```python
from build123d import *

# Parameters (mm, degrees)
SKETCH1_W                   = 38.1
SKETCH1_H                   = 25.4
BOSS_EXTRUDE1_DEPTH         = 25.4
SKETCH3_R                   = 1.5875
CUT_EXTRUDE2_DEPTH          = 25.4
F_1_4_28_TAPPED_HOLE1_D     = 5.4102
F_1_4_28_TAPPED_HOLE1_DEPTH = 17.23
F_1_4_28_TAPPED_HOLE1_TIP   = 1.625388061
SKETCH2_R                   = 3.18
CUT_EXTRUDE6_DEPTH          = 15.875
SKETCH8_R                   = 1.5875
CUT_EXTRUDE7_DEPTH          = 35.1957966
SKETCH9_W                   = 19.05
SKETCH9_H                   = 25.4
BOSS_EXTRUDE2_DEPTH         = 12.7
SKETCH12_W                  = 38.05497839
SKETCH12_H                  = 25.4
BOSS_EXTRUDE3_DEPTH         = 44.45
CUT_EXTRUDE8_START          = -44.45
SKETCH14_R                  = 1.5875
CUT_EXTRUDE8_DEPTH          = 44.45
F_1_4_28_TAPPED_HOLE2_D     = 5.4102
F_1_4_28_TAPPED_HOLE2_DEPTH = 17.23
F_1_4_28_TAPPED_HOLE2_TIP   = 1.625388061
BOSS_EXTRUDE6_DEPTH         = 34.925


with BuildPart() as part:
    # Sketch1 → Boss-Extrude1 (new body)
    with BuildSketch(Plane(origin=(0, 0, 0), x_dir=(1, 0, 0), z_dir=(0, 1, 0))):
        Rectangle(SKETCH1_W, SKETCH1_H)
    extrude(amount=BOSS_EXTRUDE1_DEPTH)

    # Sketch3 → Cut-Extrude2 (cut)
    with BuildSketch(Plane.ZY.offset(19.05)):
        with Locations((0, 12.7)):
            Circle(SKETCH3_R)
    extrude(amount=-CUT_EXTRUDE2_DEPTH, mode=Mode.SUBTRACT)

    # 1/4-28 Tapped Hole1
    with Locations(Plane.ZY.offset(19.05)):
        with Locations((0, 12.7)):
            Hole(F_1_4_28_TAPPED_HOLE1_D / 2, depth=F_1_4_28_TAPPED_HOLE1_DEPTH)
            with Locations((0, 0, -(F_1_4_28_TAPPED_HOLE1_DEPTH + F_1_4_28_TAPPED_HOLE1_TIP / 2))):  # 118° drill point
                Cone(0, F_1_4_28_TAPPED_HOLE1_D / 2, F_1_4_28_TAPPED_HOLE1_TIP, mode=Mode.SUBTRACT)

    # Sketch2 → Cut-Extrude6 (cut)
    with BuildSketch(Plane(origin=(0, 25.4, 0), x_dir=(1, 0, 0), z_dir=(0, 1, 0))):
        with Locations(Location((6.35, 0, 0), (0, 0, 270))):
            Circle(SKETCH2_R)
    extrude(amount=-CUT_EXTRUDE6_DEPTH, mode=Mode.SUBTRACT)

    # Sketch8 → Cut-Extrude7 (cut, through all)
    with BuildSketch(Plane.XZ):
        with Locations(Location((6.35, 0, 0), (0, 0, 270))):
            Circle(SKETCH8_R)
    extrude(amount=-CUT_EXTRUDE7_DEPTH, mode=Mode.SUBTRACT)

    # Sketch9 → Boss-Extrude2 (add)
    with BuildSketch(Plane.XZ):
        with Locations((-9.525, 0)):
            Rectangle(SKETCH9_W, SKETCH9_H)
    extrude(amount=BOSS_EXTRUDE2_DEPTH)

    # Sketch12 → Boss-Extrude3 (add)
    with BuildSketch(Plane.XZ.offset(12.7)):
        with Locations((-0.022510805, 0)):
            Rectangle(SKETCH12_W, SKETCH12_H)
    extrude(amount=BOSS_EXTRUDE3_DEPTH)

    # Sketch14 → Cut-Extrude8 (cut)
    with BuildSketch(Plane(origin=(0, -12.7, 0), x_dir=(1, 0, 0), z_dir=(0, 1, 0)).offset(CUT_EXTRUDE8_START)):
        with Locations(Location((6.35, 0, 0), (0, 0, 90))):
            Circle(SKETCH14_R)
    extrude(amount=CUT_EXTRUDE8_DEPTH, mode=Mode.SUBTRACT)

    # 1/4-28 Tapped Hole2
    with Locations(Plane(origin=(0, -57.15, 0), x_dir=(-1, 0, 0), z_dir=(0, -1, 0))):
        with Locations((-6.35, 0)):
            Hole(F_1_4_28_TAPPED_HOLE2_D / 2, depth=F_1_4_28_TAPPED_HOLE2_DEPTH)
            with Locations((0, 0, -(F_1_4_28_TAPPED_HOLE2_DEPTH + F_1_4_28_TAPPED_HOLE2_TIP / 2))):  # 118° drill point
                Cone(0, F_1_4_28_TAPPED_HOLE2_D / 2, F_1_4_28_TAPPED_HOLE2_TIP, mode=Mode.SUBTRACT)

    # Sketch24 → Boss-Extrude6 (add)
    with BuildSketch(Plane(origin=(0, 25.4, 0), x_dir=(1, 0, 0), z_dir=(0, 1, 0))):
        with BuildLine():
            Line((6.35, -3.302), (19.05, -3.302))
            Line((19.05, -3.302), (19.05, -12.7))
            Line((19.05, -12.7), (-19.05, -12.7))
            Line((-19.05, -12.7), (-19.05, 12.7))
            Line((-19.05, 12.7), (19.05, 12.7))
            Line((19.05, 12.7), (19.05, 3.302))
            Line((19.05, 3.302), (6.35, 3.302))
            ThreePointArc((6.35, 3.302), (3.048, 0), (6.35, -3.302))
        make_face()
    extrude(amount=BOSS_EXTRUDE6_DEPTH)


solid = part.part
```
The model under review builds one solid part; all positions refer to its coordinate system, in mm. A direction names the side the tool comes from. Round coordinates to 2 decimals unless told otherwise and drop trailing zeros. Order: outer loops, then holes, each group sorted by start corner. A loop starts at its lowest first (then second) coordinate and runs counter-clockwise, first axis right, second up. Notation, with made-up numbers: (25, 50) -> (29, 50) arc R27 ccw to (29, 86) -> close; hole circle Ø7 at (-31.75, 64). An arc over 180 degrees is marked (long way). One line per item, written item: value. Start each with the question number.
Q1. Take a section at B-B (x = 16). Write out the cut boundary in (y, z) (3 decimals).
Q2. Take a section at A-A (z = 0). Count the separate pieces of the cut face and the enclosed holes in it, and give its area (3 significant figures).
Q3. Mouldability with a two-part tool opening along X and no side actions: class faces 5 (the face through (19.05, 23, 0)), 6 (the face through (4.94, 4.7, -0.73)), 7 (the face through (8, 9.525, 1)), 8 (the face through (-19.05, 1, 0)) as released by +X, released by -X, zero draft, split by the parting line, or undercut.
Q4. Take a section at D-D (z = -10). Write out the cut boundary in (x, y) (3 decimals), and give its area (3 significant figures).
Q5. Take a section at C-C (y = -49). Write out the cut boundary in (x, z).
Q6. Wall thickness on line 1 (Y direction, x = 8.5, z = 6.5) (3 decimals); line 2 (Y direction, x = -6.25, z = 0) (3 decimals); line 3 (X direction, y = 16.25, z = 0): over which ranges is each line inside the solid? List them lowest first.
Q7. Machinability: for faces 1 (the face through (3.05, 42.62, -0.07)), 2 (the face through (0, 60.325, 0)), 3 (the face through (0, -6, 0)), 4 (the face through (1.19, 12.77, -1.586)), which of the approach directions +Z, -Z, +X, -X, +Y, -Y give a long, thin tool a straight path to every point of the face, cutting with its end or side? Answer none if there is none.
Q8. Clearance check with flat-ended pins moving along their axes: pin 1 Ø4.5 at (x, z) = (6.35, 0) entering from -Y; pin 2 Ø3.5 at (x, z) = (6.35, 0) entering from +Y (3 decimals); pin 3 Ø1.5 at (y, z) = (-22, -2.5) entering from +X (3 decimals); pin 4 Ø8.5 at (x, z) = (6.35, 0) entering from -Y. State where each tip first meets the part, or that it passes through.
Reported:
1. outline: (-57.15, -12.7) -> (-12.7, -12.7) -> (-12.7, 12.7) -> (-57.15, 12.7) -> close; (0, -12.7) -> (60.325, -12.7) -> (60.325, -3.302) -> (25.4, -3.302) -> (25.4, 3.302) -> (60.325, 3.302) -> (60.325, 12.7) -> (0, 12.7) -> close
2. separate pieces: 4
2. enclosed holes: 0
2. area: 3,250 mm2
3. face 5: released by +X
3. face 6: undercut
3. face 7: undercut
3. face 8: released by -X
4. outline: (-19.05, -57.15) -> (19.005, -57.15) -> (19.005, -12.7) -> (0, -12.7) -> (0, 0) -> (19.05, 0) -> (19.05, 60.325) -> (-19.05, 60.325) -> close
4. area: 4,230 mm2
5. outline: (-19.05, -12.7) -> (19, -12.7) -> (19, 12.7) -> (-19.05, 12.7) -> close; hole circle Ø5.41 at (6.35, 0)
6. line 1: y = -57.15 to -12.7, 0 to 60.325
6. line 2: y = -57.15 to 9.995, 15.405 to 60.325
6. line 3: x = -19.05 to 3.17, 9.53 to 19.05
7. face 1: +X, +Y
7. face 2: +Z, -Z, +X, -X, +Y
7. face 3: +Z, -Z, +X
7. face 4: -X
8. pin 1: stops at y = -39.65
8. pin 2: stops at y = 9.525
8. pin 3: stops at x = 19.005
8. pin 4: stops at y = -57.15
